```python
from build123d import *

# Parameters (mm, degrees)
SKETCH_1_W          = 70
SKETCH_1_H          = 20
EXTRUDE_1_DEPTH     = 5
SKETCH_2_R          = 1.575
CUT_EXTRUDE_1_DEPTH = 73.972597597


with BuildPart() as part:
    # 草图1 → 凸台-拉伸1 (new body)
    with BuildSketch(Plane.XY):
        with Locations((35, -10)):
            Rectangle(SKETCH_1_W, SKETCH_1_H)
    extrude(amount=EXTRUDE_1_DEPTH)

    # 草图2 → 切除-拉伸1 (cut, through all)
    with BuildSketch(Plane.XY.offset(5)):
        with Locations((5, -5)):
            Circle(SKETCH_2_R)
        with Locations(Location((5, -15, 0), (0, 0, 180))):
            Circle(SKETCH_2_R)
        with Locations((15, -15)):
            Circle(SKETCH_2_R)
        with Locations(Location((15, -5, 0), (0, 0, 180))):
            Circle(SKETCH_2_R)
        with Locations((55, -5)):
            Circle(SKETCH_2_R)
        with Locations(Location((55, -15, 0), (0, 0, 180))):
            Circle(SKETCH_2_R)
        with Locations((65, -15)):
            Circle(SKETCH_2_R)
        with Locations(Location((65, -5, 0), (0, 0, 180))):
            Circle(SKETCH_2_R)
    extrude(amount=-CUT_EXTRUDE_1_DEPTH, mode=Mode.SUBTRACT)


solid = part.part
```
Read the model definition and answer for the solid it produces. Units are mm, in the model's axes. Round coordinates to 2 decimals unless told otherwise and drop trailing zeros. Write each loop counter-clockwise with the first axis right and the second up, starting at its lowest first coordinate (ties: lowest second). Pieces come first, ordered by that corner, then holes. Notation, with made-up numbers: (-25.5, -29.5) -> (-21.5, -29.5) arc R25 cw to (-21.5, -17.5) -> close; hole circle Ø10 at (1, -1.5). An arc over 180 degrees is marked (long way). Answer in a Markdown table with one row per item. Add a question column.
1) Consider line 1 (Y direction, x = 65, z = 2) (3 decimals); line 2 (X direction, y = -4.5, z = 2.25). Determine where each line is inside the solid, lowest interval first.
2) Find section C-C, the plane y = -15. Determine the outline of the cut face in (x, z) (3 decimals).
3) Find section A-A, the plane x = 15. Determine the outline of the cut face in (y, z) (3 decimals).
4) Determine the mould class of faces 1 (the face through (35, -10, 0)), 2 (the face through (0, -10, 2)), 3 (the face through (3.839, -3.936, 2.535)), 4 (the face through (63.498, -5.473, 2.535)) for opening direction X: pulls with the +X half, pulls with the -X half, needs draft (parallel to the pull), parting line crosses it, or undercut.
5) Find section B-B, the plane z = 3.1. State how many separate pieces and enclosed holes the cut face has, and give its area (3 significant figures).
6) Given P1, Ø3.5, axis at x = 5, y = -15, coming from the -Z side; P2, Ø2.5, axis at x = 55, y = -15, coming from the +Z side, each flat-ended and moving along its own axis, determine where each tip first touches the part or whether it passes through.
Findings below:
| question | item | result |
|---|---|---|
| 1 | line 1 | -20 to -16.575, -13.425 to -6.575, -3.425 to 0 |
| 1 | line 2 | 0 to 3.51, 6.49 to 13.51, 16.49 to 53.51, 56.49 to 63.51, 66.49 to 70 |
| 2 | outline | (0, 0) -> (3.425, 0) -> (3.425, 5) -> (0, 5) -> close; (6.575, 0) -> (13.425, 0) -> (13.425, 5) -> (6.575, 5) -> close; (16.575, 0) -> (53.425, 0) -> (53.425, 5) -> (16.575, 5) -> close; (56.575, 0) -> (63.425, 0) -> (63.425, 5) -> (56.575, 5) -> close; (66.575, 0) -> (70, 0) -> (70, 5) -> (66.575, 5) -> close |
| 3 | outline | (-20, 0) -> (-16.575, 0) -> (-16.575, 5) -> (-20, 5) -> close; (-13.425, 0) -> (-6.575, 0) -> (-6.575, 5) -> (-13.425, 5) -> close; (-3.425, 0) -> (0, 0) -> (0, 5) -> (-3.425, 5) -> close |
| 4 | face 1 | needs draft |
| 4 | face 2 | pulls with the -X half |
| 4 | face 3 | undercut |
| 4 | face 4 | undercut |
| 5 | separate pieces | 1 |
| 5 | enclosed holes | 8 |
| 5 | area | 1,340 mm² |
| 6 | P1 | z = 0 |
| 6 | P2 | through |
